Autodesk Inventor part; units mm, degrees
ref_plane "YZ Plane" through (0, 0, 0) normal (1, 0, 0) x (0, 1, 0)
ref_plane "XZ Plane" through (0, 0, 0) normal (0, 1, 0) x (-1, 0, 0)
ref_plane "XY Plane" through (0, 0, 0) normal (0, 0, 1) x (1, 0, 0)
sketch "Эскиз1" plane through (0, 0, 0) normal (0, 0, 1) x (1, 0, 0)
  line L0 (12.5, 7) -> (-12.5, 7)
  line L1 (-12.5, 7) -> (-12.5, -7)
  line L2 (-12.5, -7) -> (12.5, -7)
  line L3 (12.5, -7) -> (12.5, 7)
  line L4 (12.5, 7) -> (-12.5, -7) construction
  line L5 (-12.5, 7) -> (12.5, -7) construction
  line L6 (-16.5, 13) -> (12.5, 13)
  line L7 (11.5, 13) -> (11.5, -10.7) construction
  line L8 (11.5, -10.7) -> (12.5, -10.7) construction
  line L9 (-16.5, -10.7) -> (-16.5, 13)
  line L10 (12.5, -7) -> (12.5, -10.7)
  line L11 (12.5, 7) -> (12.5, 13)
  line L12 (12.5, 13) -> (11.5, 13) construction
  line L13 (12.5, -10.7) -> (-16.5, -10.7)
  point P0 (0, 0)
  dimension "d0" = 25
  dimension "d1" = 14
  dimension "d2" = 6
  dimension "d11" = 3.7
extrude "Выдавливание1" add sketch "Эскиз1" along normal blind 50 contours L0 L1 L2 L10 L13 L9 L6 L11
sketch "Эскиз2" plane through (-16.5, -10.7, 0) normal (-1, 0, 0) x (0, 0, 1)
  line L0 (0, 23.7) -> (0, 0) construction
  line L1 (0, 0) -> (50, 0) construction
  line L2 (50, 23.7) -> (50, 0) construction
  line L3 (0, 23.7) -> (50, 23.7) construction
  line L4 (45, 19.7) -> (5, 19.7)
  line L5 (5, 19.7) -> (5, 4)
  line L6 (45, 4) -> (45, 19.7)
  line L7 (45, 19.7) -> (5, 4) construction
  line L8 (5, 19.7) -> (45, 4) construction
  line L9 (0, 23.7) -> (50, 23.7)
  line L10 (50, 0) -> (50, 3.7)
  line L11 (0, 23.7) -> (50, 0) construction
  line L12 (5, 3.7) -> (45, 3.7)
  line L13 (5, 4) -> (5, 3.7)
  line L14 (0, 3.7) -> (50, 3.7)
  line L15 (45, 4) -> (45, 3.7)
  point P0 (0, 10.7)
  point P1 (25, 11.85)
  dimension "d5" = 40
  dimension "d6" = 4
  dimension "d12" = 3.7
extrude "Выдавливание2" cut sketch "Эскиз2" against normal blind 4
sketch "Эскиз4" plane through (-16.5, -10.7, 0) normal (0, -1, 0) x (1, 0, 0)
  circle A0 centre (2.5, 32.95) radius 1.5 construction
  circle A1 centre (2.5, 16.95) radius 1.5 construction
  circle A2 centre (17.5, 32.95) radius 1.5 construction
  circle A3 centre (2.5, 16.95) radius 1.5 construction
  circle A4 centre (17.5, 16.95) radius 1.5 construction
  circle A5 centre (2.5, 32.95) radius 1.6
  circle A6 centre (17.5, 32.95) radius 1.6
  circle A7 centre (17.5, 16.95) radius 1.6
  circle A8 centre (2.5, 16.95) radius 1.6
  dimension "d19" = 3.2
  dimension "d20" = 3.2
  dimension "d21" = 3.2
  dimension "d22" = 3.2
extrude "Выдавливание3" cut sketch "Эскиз4" against normal blind 4
sketch "Эскиз6" plane through (-16.5, 13, 0) normal (0, 1, 0) x (1, 0, 0)
  circle A0 centre (9.8, -9.6796) radius 6 construction
  line L0 (15.8, -9.6796) -> (15.8, -27.7296) construction
  circle A1 centre (21.8, -6) radius 6 construction
  circle A2 centre (21.8, -6) radius 2.1
  line L1 (29, -25) -> (0, -25) construction
  circle A3 centre (21.8, -44) radius 2.1
  dimension "d13" = 12
  dimension "d14" = 12
  dimension "d15" = 4.2
extrude "Выдавливание4" cut sketch "Эскиз6" against normal blind 5
properties part number "креп_центр_ролик"
The listing builds one solid part. Answer for the finished solid, in the listing's coordinates (mm). A direction names the side the tool comes from. Give positions to 0.01 mm unless a question says otherwise; leave off trailing zeros. Order: outer loops, then holes, each group sorted by start corner. A loop starts at its lowest first (then second) coordinate and runs counter-clockwise, first axis right, second up. Notation, with made-up numbers: (13, -24.75) - (30, -24.75) arc R31 cw to (30, 11.25) - close; hole circle Ø5 at (5, 81.5). An arc over 180 degrees is marked (long way). Use one line per item in the form item = value. Start each with the question number.
(1) The mould has two halves that part along Z. Classify faces 1 (the flat face through (0, 7, 25)), 2 (the cylindrical face through (-15.6, -8.9, 17)), 3 (the flat face through (-5, 9, 50)): released by +Z, released by -Z, zero draft, split by the parting line, or undercut.
(2) A cutting plane is placed at D-D, the plane x = -14. Write down the section's boundary in (y, z), then the cut area to 3 significant figures.
(3) Flat-ended cylindrical pins translate along their axes: pin 1 Ø1.5 at (y, z) = (-2, 3.5) entering from +X; pin 2 Ø2 at (y, z) = (7.5, 25.5) entering from -X; pin 3 Ø3.5 at (x, z) = (5, 44) entering from +Y. Find the tip coordinate at first contact, or state that the pin passes through.
(4) For faces 4 (the flat face through (5, 8, 6)), 5 (the flat face through (-12.5, 0, 2)), 6 (the cylindrical face through (0.65, -8.88, 15.39)), 7 (the flat face through (-5, 9, 0)), determine the directions among +Z, -Z, +X, -X, +Y, -Y from which every point of the face is accessible in a straight line to the end or side of a thin tool.
(5) A cutting plane is placed at A-A, the plane z = 16.95. Write down the section's boundary in (x, y), then the cut area to 3 significant figures.
(6) A cutting plane is placed at B-B, the plane x = 1. Write down the section's boundary in (y, z).
(7) A cutting plane is placed at C-C, the plane y = 4.75. Write down the section's boundary in (x, z).
(8) Consider line 1 (Z direction, x = 5.3, y = 11.3); line 2 (Y direction, x = 3, z = 16); line 3 (Z direction, x = -13, y = -5.25). Determine where each line is inside the solid, lowest interval first. Write a range as from..to.
Ans:
q1.face_1 = zero draft
q1.face_2 = undercut
q1.face_3 = released by +Z
q2.outline = (-10.7, 0) - (13, 0) - (13, 50) - (-10.7, 50) - (-10.7, 34.55) - (-7, 34.55) - (-7, 45) - (9, 45) - (9, 5) - (-7, 5) - (-7, 15.35) - (-10.7, 15.35) - close; (-10.7, 18.55) - (-7, 18.55) - (-7, 31.35) - (-10.7, 31.35) - close
q2.area = 521 mm^2
q3.pin_1 = -12.5
q3.pin_2 = -12.5
q3.pin_3 = 8
q4.face_4 = +Y
q4.face_5 = +Z, -Z, +X
q4.face_6 = -Y
q4.face_7 = -Z, +X, -X, +Y, -Y
q5.outline = (-16.5, -10.7) - (-15.6, -10.7) - (-15.6, -7) - (-16.5, -7) - close; (-16.5, 9) - (-12.5, 9) - (-12.5, 7) - (12.5, 7) - (12.5, 13) - (-16.5, 13) - close; (-12.4, -10.7) - (-0.6, -10.7) - (-0.6, -7) - (-12.4, -7) - close; (2.6, -10.7) - (12.5, -10.7) - (12.5, -7) - (2.6, -7) - close
q5.area = 250 mm^2
q6.outline = (-10.7, 0) - (-7, 0) - (-7, 15.35) - (-10.7, 15.35) - close; (-10.7, 18.55) - (-7, 18.55) - (-7, 31.35) - (-10.7, 31.35) - close; (-10.7, 34.55) - (-7, 34.55) - (-7, 50) - (-10.7, 50) - close; (7, 0) - (13, 0) - (13, 50) - (7, 50) - close
q7.outline = (-16.5, 0) - (-12.5, 0) - (-12.5, 5) - (-16.5, 5) - close; (-16.5, 45) - (-12.5, 45) - (-12.5, 50) - (-16.5, 50) - close
q8.line_1 = 0..3.9, 8.1..41.9, 46.1..50
q8.line_2 = -10.7..-7, 7..13
q8.line_3 = 0..5, 45..50
